Source: three-view drawing plus pictorial views. Frame: mm from the lowest corner of the part. Round coordinates to 2 decimals unless told otherwise and drop trailing zeros. Loops run counter-clockwise (first coordinate to the right, second up) from the corner with the lowest first, then second, coordinate; pieces in that order, holes last. Notation, with made-up numbers: (4.5, -38.5) -> (34.5, -38.5) arc R25 cw to (34.5, -16.5) -> close; hole circle Ø7 at (-7.75, 31.5). An arc over 180 degrees is marked (long way). Answer in a Markdown table with one row per item. Add a question column.
Q1. Section B-B, the plane x = 42.95. Output: boundary loops of the cut face in (y, z), and give its area (3 significant figures).
Q2. Ray query, L1, parallel to X at y = 54.5, z = 3.1; L2, parallel to Y at x = 217.05, z = 1.9; L3, parallel to Y at x = 10, z = 1.35. Return the intervals inside material, ascending. Write a range as from..to.
Q3. Section C-C, the plane z = 3.3. Output: boundary loops of the cut face in (x, y).
Q4. Section D-D, the plane x = 119.5. Output: boundary loops of the cut face in (y, z).
Q5. Section A-A, the plane y = 55. Output: boundary loops of the cut face in (x, z).
Q6. Pin query (flat end, axial travel): pin 1 (2 mm diameter, centred on x = 115, z = 1, fed in from -Y); pin 2 (2 mm diameter, centred on y = 8.5, z = 3, fed in from +X); pin 3 (1.2 mm diameter, centred on y = 6.5, z = 3, fed in from +X). Return the tip coordinate at first contact, or that it passes through.
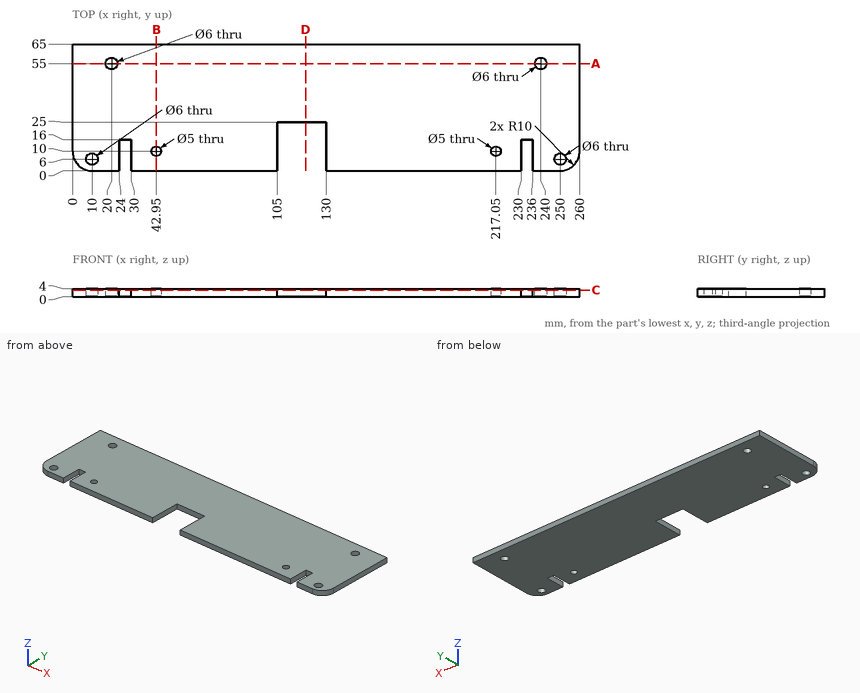
Answer block:
| question | item | result |
|---|---|---|
| 1 | outline | (0, 0) -> (7.5, 0) -> (7.5, 4) -> (0, 4) -> close; (12.5, 0) -> (65, 0) -> (65, 4) -> (12.5, 4) -> close |
| 1 | area | 240 mm^2 |
| 2 | L1 | 0..17.04, 22.96..237.04, 242.96..260 |
| 2 | L2 | 0..7.5, 12.5..65 |
| 2 | L3 | 0..3, 9..65 |
| 3 | outline | (0, 10) arc R10 ccw to (10, 0) -> (24, 0) -> (24, 16) -> (30, 16) -> (30, 0) -> (105, 0) -> (105, 25) -> (130, 25) -> (130, 0) -> (230, 0) -> (230, 16) -> (236, 16) -> (236, 0) -> (250, 0) arc R10 ccw to (260, 10) -> (260, 65) -> (0, 65) -> close; hole circle Ø6 at (10, 6); hole circle Ø6 at (20, 55); hole circle Ø5 at (42.95, 10); hole circle Ø5 at (217.05, 10); hole circle Ø6 at (240, 55); hole circle Ø6 at (250, 6) |
| 4 | outline | (25, 0) -> (65, 0) -> (65, 4) -> (25, 4) -> close |
| 5 | outline | (0, 0) -> (17, 0) -> (17, 4) -> (0, 4) -> close; (23, 0) -> (237, 0) -> (237, 4) -> (23, 4) -> close; (243, 0) -> (260, 0) -> (260, 4) -> (243, 4) -> close |
| 6 | pin 1 | y = 25 |
| 6 | pin 2 | x = 259.99 |
| 6 | pin 3 | x = 259.57 |
